Part model, mm, in its own coordinate system. Round coordinates to 2 decimals unless told otherwise and drop trailing zeros. Order: outer loops, then holes, each group sorted by start corner. A loop starts at its lowest first (then second) coordinate and runs counter-clockwise, first axis right, second up. Notation, with made-up numbers: (12.5, 12.25) -> (17.5, 12.25) arc R18 cw to (17.5, 35.25) -> close; hole circle Ø8 at (20.5, 53). An arc over 180 degrees is marked (long way). Answer as a JSON object with one key per item and string values. Group by question number.
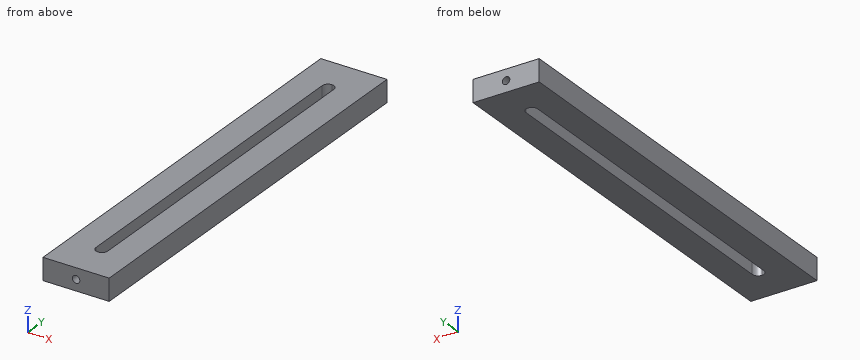
Autodesk Inventor part; units mm, degrees
ref_plane "YZ Plane" through (0, 0, 0) normal (1, 0, 0) x (0, 1, 0)
ref_plane "XZ Plane" through (0, 0, 0) normal (0, 1, 0) x (-1, 0, 0)
ref_plane "XY Plane" through (0, 0, 0) normal (0, 0, 1) x (1, 0, 0)
sketch "Sketch1" plane through (0, 0, 0) normal (0, 0, 1) x (1, 0, 0)
  line L0 (-9.525, -60.325) -> (9.525, -60.325)
  line L1 (9.525, -60.325) -> (9.525, 60.325)
  line L2 (9.525, 60.325) -> (-9.525, 60.325)
  line L3 (-9.525, 60.325) -> (-9.525, -60.325)
  line L4 (-9.525, -60.325) -> (9.525, 60.325) construction
  line L5 (9.525, -60.325) -> (-9.525, 60.325) construction
  point P0 (0, 0)
  dimension "d0" = 19.05
  dimension "d1" = 120.65
extrude "Extrusion1" add sketch "Sketch1" along normal blind 6.35
sketch "Sketch2" plane through (0, 0, 6.35) normal (0, 0, 1) x (1, 0, 0)
  line L0 (1.6891, -50.8) -> (-1.6891, -50.8)
  line L1 (-1.6891, -50.8) -> (-1.6891, 50.8)
  line L2 (-1.6891, 50.8) -> (1.6891, 50.8)
  line L3 (1.6891, 50.8) -> (1.6891, -50.8)
  line L4 (1.6891, -50.8) -> (-1.6891, 50.8) construction
  line L5 (-1.6891, -50.8) -> (1.6891, 50.8) construction
  point P0 (0, 0)
  dimension "d4" = 3.3782
  dimension "d5" = 101.6
extrude "Extrusion2" cut sketch "Sketch2" against normal through all
fillet "Fillet1" radius 1.6891 4 edges at (-1.6891, -50.8, 3.175) (1.6891, -50.8, 3.175) (-1.6891, 50.8, 3.175) (1.6891, 50.8, 3.175)
sketch "Sketch4" plane through (-9.525, -60.325, 0) normal (0, -1, 0) x (1, 0, 0)
  line L0 (0, 0) -> (19.05, 0)
  line L1 (19.05, 0) -> (19.05, 6.35)
  line L2 (0, 6.35) -> (19.05, 6.35)
  line L3 (0, 0) -> (0, 6.35)
  point P0 (9.525, 0)
  point P1 (9.525, 3.175)
  dimension "d16" = 3.175
  dimension "d17" = 9.525
hole "Hole2" at (0, -60.325, 3.175) direction (0, 1, 0) diameter 2.156 depth 8.865 tip angle 118
mirror "Mirror1" about plane through (0, 0, 0) normal (0, 1, 0) of "Hole2"
equation "\"d0\" = sensorHolderDepth"
equation "\"d1\" = -internalAcrylicThickness + height"
equation "\"d2\" = acrylicThickness"
equation "\"d5\" = height - 4 * acrylicThickness"
equation "\"d6\" = acrylicThickness"
equation "\"acrylicThickness\" = 6.35"
equation "\"height\" = 127"
equation "\"sensorHolderDepth\" = 19.05"
equation "\"frameAcrylicThickness\" = 9.525"
equation "\"internalAcrylicThicnkess\" = 6.35"
equation "\"width\" = 127"
equation "\"depth\" = 273.05"
equation "\"mirrorAngle\" = 5deg"
equation "\"detectorWidth\" = 52"
equation "\"detectorHeight\" = 52"
equation "\"mirrorThickness\" = 3.175"
equation "\"fresnelThickness\" = 0.1"
equation "\"focalLength\" = 76.2"
equation "\"ior\" = 1.49"
equation "\"centerThickness\" = 1.524"
equation "\"fresnelAngle\" = 90deg"
equation "\"fresnelEffectiveDiameter\" = 152.4"
equation "\"oRingWidth\" = 1.5875"
equation "\"internalAcrylicThickness\" = 6.35"
equation "\"aerogelClearence\" = 3.175"
equation "\"backplaneHoleOffsett\" = 6.35"
equation "\"backplanePCBHeight\" = 76.2"
equation "\"backplanePCBWidth\" = 76.2"
equation "\"backplanePostionOffsett\" = 12.7"
equation "\"moduleSlotClearence\" = 0.79375"
properties part number "verticalSupourt" material "ABS Plastic"
Q1. Band-saw the part on A-A (y = 3.5). List the corners of the cut face in (x, z) (3 decimals).
Q2. Wall check: line 1 (X direction, y = -48, z = 0.75) (3 decimals); line 2 (Z direction, x = 0, y = -58.25); line 3 (Y direction, x = 0, z = 0.5) (3 decimals). Give the ranges that are in metal, low to high. Write a range as [from, to].
Q3. Drop a flat-ended pin along its axis: pin 1 Ø1.7 at (x, z) = (0, 3.175) entering from -Y. Give the stop position or say it passes through.
Completed:
{
 "1": {"outline": "(-9.525, 0) -> (-1.689, 0) -> (-1.689, 6.35) -> (-9.525, 6.35) -> close; (1.689, 0) -> (9.525, 0) -> (9.525, 6.35) -> (1.689, 6.35) -> close"},
 "2": {"line 1": "[-9.525, -1.689], [1.689, 9.525]", "line 2": "[0, 2.1], [4.25, 6.35]", "line 3": "[-60.325, -50.8], [50.8, 60.325]"},
 "3": {"pin 1": "y = -51.32"}
}
